```python
from build123d import *

# Parameters (mm, degrees)
SKETCH1_W           = 8.8
SKETCH1_H           = 8.8
BOSS_EXTRUDE1_DEPTH = 54.75
SKETCH2_R           = 1.95
CUT_EXTRUDE1_DEPTH  = 8
CUT_EXTRUDE2_REACH  = 57.627
SKETCH3_R           = 1.95
CHAMFER1_SIZE       = 0.5
CHAMFER2_SIZE       = 0.25


with BuildPart() as part:
    # Sketch1 → Boss-Extrude1 (new, symmetric)
    with BuildSketch(Plane.XY):
        Rectangle(SKETCH1_W, SKETCH1_H)
    extrude(amount=BOSS_EXTRUDE1_DEPTH, both=True)

    # Sketch2 → Cut-Extrude1 (cut)
    with BuildSketch(Plane.XY.offset(54.75)):
        Circle(SKETCH2_R)
    cut_extrude1 = extrude(amount=-CUT_EXTRUDE1_DEPTH, mode=Mode.SUBTRACT)

    # Mirror1: Cut-Extrude1 across plane
    add(cut_extrude1.mirror(Plane.XY), mode=Mode.SUBTRACT)

    # Sketch3 → Cut-Extrude2 (cut, up to next)
    with BuildSketch(Plane(origin=(4.4, 0, 0), x_dir=(0, 0, -1), z_dir=(1, 0, 0)), mode=Mode.PRIVATE) as cut_extrude2_sk1:
        with Locations((-30, 0)):
            Circle(SKETCH3_R)
    cut_extrude2_tool1 = extrude(cut_extrude2_sk1.sketch, amount=-CUT_EXTRUDE2_REACH, mode=Mode.PRIVATE) & part.part
    # Sketch3 → Cut-Extrude2 (cut, up to next)
    with BuildSketch(Plane(origin=(4.4, 0, 0), x_dir=(0, 0, -1), z_dir=(1, 0, 0)), mode=Mode.PRIVATE) as cut_extrude2_sk2:
        with Locations((30, 0)):
            Circle(SKETCH3_R)
    cut_extrude2_tool2 = extrude(cut_extrude2_sk2.sketch, amount=-CUT_EXTRUDE2_REACH, mode=Mode.PRIVATE) & part.part
    add(cut_extrude2_tool1.solids().sort_by_distance((4.4, 0, 30))[0], mode=Mode.SUBTRACT)
    add(cut_extrude2_tool2.solids().sort_by_distance((4.4, 0, -30))[0], mode=Mode.SUBTRACT)

    # Chamfer1
    chamfer1_edges = [part.edges().sort_by_distance(p)[0] for p in [
        (-1.95, 0, 54.75),
        (-1.95, 0, -54.75),
        (4.4, 0, 31.95),
        (-4.4, 0, 31.95),
        (4.4, 0, -28.05),
        (-4.4, 0, -28.05),
    ]]
    chamfer(chamfer1_edges, length=CHAMFER1_SIZE)

    # Chamfer2
    chamfer2_edges = [part.edges().sort_by_distance(p)[0] for p in [
        (-4.4, 0, 54.75),
        (0, -4.4, 54.75),
        (4.4, 0, 54.75),
        (0, -4.4, -54.75),
        (-4.4, 0, -54.75),
        (0, 4.4, -54.75),
        (4.4, 0, -54.75),
        (4.4, -4.4, 0),
        (-4.4, -4.4, 0),
        (-4.4, 4.4, 0),
        (4.4, 4.4, 0),
        (0, 4.4, 54.75),
    ]]
    chamfer(chamfer2_edges, length=CHAMFER2_SIZE)


solid = part.part
```
CAD build for the part. Positions are in the model's coordinates, mm. A direction names the side the tool comes from. Round coordinates to 2 decimals unless told otherwise and drop trailing zeros. Order: outer loops, then holes, each group sorted by start corner. A loop starts at its lowest first (then second) coordinate and runs counter-clockwise, first axis right, second up. Notation, with made-up numbers: (-12, -26) - (25, -26) arc R21 ccw to (25, 5) - close; hole circle Ø10 at (49.25, 51.5). An arc over 180 degrees is marked (long way). Use CSV: the item, a comma, the result in double quotes. Start each with the question number.
1) Saw through at A-A (z = -30). List the corners of the cut face in (x, y).
2) Tool access for faces 1 (the cylindrical face through (-1.437, 1.318, -50.552)), 2 (the flat face through (0, 0, 46.75)), 3 (the flat face through (0, 4.4, 1)): list every direction of +Z, -Z, +X, -X, +Y, -Y with a clear straight run to the whole face (end or side of a thin tool).
3) Pin check, flat tips, straight feed: pin 1 Ø4.5 at (x, y) = (0, 0) entering from +Z; pin 2 Ø3 at (x, y) = (0, 0) entering from -Z. Stop position of each tip, or through.
4) Wall check: L1, parallel to Y at x = -1, z = -30; L2, parallel to Z at x = -3.75, y = -1.25; L3, parallel to Z at x = 0.5, y = -1.75. Give the ranges that are in metal, low to high. Write a range as [from, to].
5) Saw through at B-B (x = 0). List the corners of the cut face in (y, z).
6) Saw through at C-C (y = 0). Count the separate pieces of the cut face and the enclosed holes in it, and give its area (3 significant figures).
7) Two-plate mould, pull along Z, no slides. Class faces 4 (the flat face through (0, -4.4, 1)), 5 (the flat face through (0, 0, -46.75)), 6 (the cylindrical face through (0.055, 1.644, -31.048)): pulls with the +Z half, pulls with the -Z half, needs draft (parallel to the pull), parting line crosses it, or undercut.
Values follow:
1,outline,"(-4.4, -4.15) - (-4.15, -4.4) - (4.15, -4.4) - (4.4, -4.15) - (4.4, -2.45) - (3.9, -1.95) - (-3.9, -1.95) - (-4.4, -2.45) - close; (-4.4, 2.45) - (-3.9, 1.95) - (3.9, 1.95) - (4.4, 2.45) - (4.4, 4.15) - (4.15, 4.4) - (-4.15, 4.4) - (-4.4, 4.15) - close"
2,face 1,"-Z"
2,face 2,"+Z"
2,face 3,"+Z, -Z, +X, -X, +Y"
3,pin 1,"stops at z = 54.55"
3,pin 2,"stops at z = -46.75"
4,L1,"y = [-4.4, -1.95], [1.95, 4.4]"
4,L2,"z = [-54.75, -31.5], [-28.5, 28.5], [31.5, 54.75]"
4,L3,"z = [-46.75, -30.86], [-29.14, 29.14], [30.86, 46.75]"
5,outline,"(-4.4, -54.5) - (-4.15, -54.75) - (-2.45, -54.75) - (-1.95, -54.25) - (-1.95, -46.75) - (1.95, -46.75) - (1.95, -54.25) - (2.45, -54.75) - (4.15, -54.75) - (4.4, -54.5) - (4.4, 54.5) - (4.15, 54.75) - (2.45, 54.75) - (1.95, 54.25) - (1.95, 46.75) - (-1.95, 46.75) - (-1.95, 54.25) - (-2.45, 54.75) - (-4.15, 54.75) - (-4.4, 54.5) - close; hole circle Ø3.9 at (0, -30); hole circle Ø3.9 at (0, 30)"
6,separate pieces,"3"
6,enclosed holes,"0"
6,area,"831 mm2"
7,face 4,"needs draft"
7,face 5,"pulls with the -Z half"
7,face 6,"undercut"
